Study the drawing (mm; zero at the part's minimum x, y, z) and answer. Coordinates: 2 decimals unless noted, no trailing zeros. Loops run counter-clockwise (first coordinate to the right, second up) from the corner with the lowest first, then second, coordinate; pieces in that order, holes last. Notation, with made-up numbers: (55, -8.5) - (106, -8.5) arc R24 cw to (106, 15.5) - close; hole circle Ø8 at (32, 50). An arc over 180 degrees is marked (long way). Use one line per item in the form item = value.
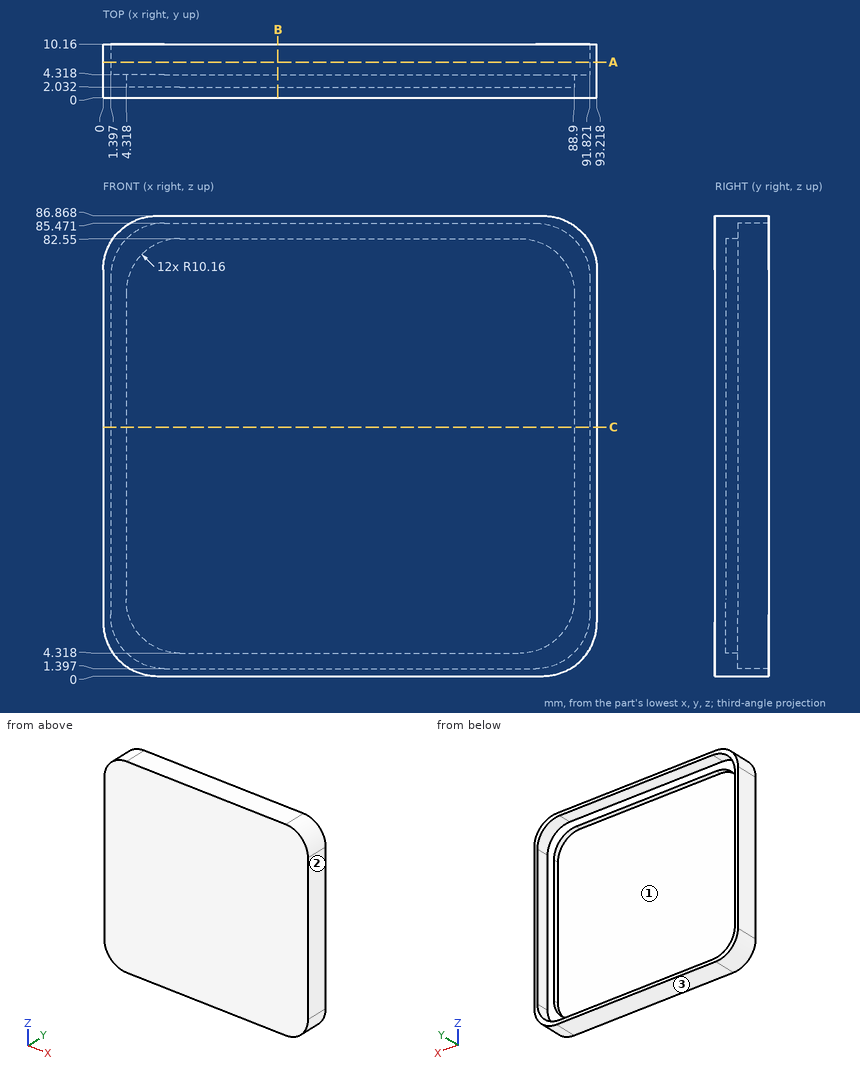
Item 1: The part is cut by section A-A on y = 6.75. Give the vertices of the cut face in (x, z).
Results below:
outline = (0, 10.16) arc R10.16 ccw to (10.16, 0) - (83.06, 0) arc R10.16 ccw to (93.22, 10.16) - (93.22, 76.71) arc R10.16 ccw to (83.06, 86.87) - (10.16, 86.87) arc R10.16 ccw to (0, 76.71) - close; hole (1.4, 11.56) arc R10.16 ccw to (11.56, 1.4) - (81.66, 1.4) arc R10.16 ccw to (91.82, 11.56) - (91.82, 75.31) arc R10.16 ccw to (81.66, 85.47) - (11.56, 85.47) arc R10.16 ccw to (1.4, 75.31) - close
Item 2: This flat-tipped pin is pushed along its axis until it touches: P1, Ø2, axis at x = 28, z = 34, coming from the +Y side. Where does it stop, or does it pass through?
Results below:
P1 = 2.03
Item 3: For a pull along X with two mould halves and no side action, classify the marked faces 1, 2 and 3 as +X half, -X half, draft (parallel to the pull), parting line (faces both ways), or undercut.
Results below:
face_1 = undercut
face_2 = +X half
face_3 = draft
Item 4: Find the intervals of material crossed by L1, parallel to Z at x = 26, y = 4.25; L2, parallel to Z at x = 26.5, y = 9.25; L3, parallel to X at y = 4, z = 23, in increasing order.
Results below:
L1 = 0 to 4.32, 82.55 to 86.87
L2 = 0 to 1.4, 85.47 to 86.87
L3 = 0 to 4.32, 88.9 to 93.22
Item 5: The part is cut by section C-C on z = 47. Give the vertices of the cut face in (x, y).
Results below:
outline = (0, 0) - (93.22, 0) - (93.22, 10.16) - (91.82, 10.16) - (91.82, 4.32) - (88.9, 4.32) - (88.9, 2.03) - (4.32, 2.03) - (4.32, 4.32) - (1.4, 4.32) - (1.4, 10.16) - (0, 10.16) - close
Item 6: The part is cut by section B-B on x = 33. Give the vertices of the cut face in (y, z).
Results below:
outline = (0, 0) - (10.16, 0) - (10.16, 1.4) - (4.32, 1.4) - (4.32, 4.32) - (2.03, 4.32) - (2.03, 82.55) - (4.32, 82.55) - (4.32, 85.47) - (10.16, 85.47) - (10.16, 86.87) - (0, 86.87) - close
